CAD build for the part. Positions are in the model's coordinates, mm. A direction names the side the tool comes from. Give positions to 0.01 mm unless a question says otherwise; leave off trailing zeros. Order: outer loops, then holes, each group sorted by start corner. A loop starts at its lowest first (then second) coordinate and runs counter-clockwise, first axis right, second up.
Item 1: Wall check: L1, parallel to X at y = 3.6, z = -24; L2, parallel to X at y = 0.4, z = 17; L3, parallel to X at y = 3.6, z = -6. Give the ranges that are in metal, low to high.
Item 2: Flat gauge pins, fed straight in: P1, Ø2, axis at x = -6, y = 2.5, coming from the +Z side; P2, Ø1, axis at x = -26, y = 0.5, coming from the +Z side (3 decimals). Where does each tip first touch, or does it go through?
Item 3: Band-saw the part on C-C on y = 2.85. Give the cut face in (x, z) (3 decimals), plus the area to 3 significant figures.
Item 4: Band-saw the part on D-D on z = 23.5. Give the cut face in (x, y).
Item 5: Which spindle directions (+Z, -Z, +X, -X, +Y, -Y) get a long thin tool onto all of the face, cutting with end or side? Do faces 5 (the flat face through (-42, 2, 26.725)), 6 (the flat face through (-31, 2, 22.225)), 7 (the flat face through (36, 2, -22.225)), 8 (the flat face through (24, 2, 0)), 9 (the flat face through (0, 2, -26.725)). Say none if no direction does.
Item 6: Two-plate mould, pull along X, no slides. Class faces 1 (the flat face through (-1, 4.5, -6)), 2 (the flat face through (-45, 2, 0)), 3 (the flat face through (40, 2, 24)), 4 (the flat face through (-40, 2, -25)): released by +X, released by -X, zero draft, split by the parting line, or undercut.
Item 7: Band-saw the part on B-B on x = 24. Give the cut face in (y, z) (3 decimals).
Item 8: Band-saw the part on A-A on z = -15. Give the cut face in (x, y), plus the area to 4 significant figures.
```python
from build123d import *

# Parameters (mm, degrees)
SKETCH1_W           = 4.5
SKETCH1_H           = 20
BOSS_EXTRUDE1_DEPTH = 4.5
SKETCH2_W           = 44.2
SKETCH2_H           = 19.225
CUT_EXTRUDE1_DEPTH  = 5.5
SKETCH3_W           = 65
SKETCH3_H           = 4.5
BOSS_EXTRUDE2_DEPTH = 4.5


with BuildPart() as part:
    # Sketch1 → Boss-Extrude1 (new body)
    with BuildSketch(Plane(origin=(0, 0, 0), x_dir=(1, 0, 0), z_dir=(0, 1, 0))):
        Polygon((-40, -22.225), (-40, -26.725), (-45, -26.725), (-45, 26.725), (-40, 26.725), (-40, 22.225), (0, 22.225), (0, -22.225), align=None)
        with Locations((-24.35, 10)):
            Rectangle(SKETCH1_W, SKETCH1_H, mode=Mode.SUBTRACT)
    boss_extrude1 = extrude(amount=BOSS_EXTRUDE1_DEPTH)

    # Mirror1: Boss-Extrude1 across plane
    add(boss_extrude1.mirror(Plane(origin=(0, 4.5, -22.225), x_dir=(0, 0, 1), z_dir=(-1, 0, 0))))

    # Sketch2 → Cut-Extrude1 (cut, through all)
    with BuildSketch(Plane(origin=(0, 4.5, 0), x_dir=(1, 0, 0), z_dir=(0, 1, 0))):
        with Locations((0, -12.6125)):
            Rectangle(SKETCH2_W, SKETCH2_H)
    extrude(amount=-CUT_EXTRUDE1_DEPTH, mode=Mode.SUBTRACT)

    # Sketch3 → Boss-Extrude2 (add)
    with BuildSketch(Plane(origin=(0, 4.5, 0), x_dir=(1, 0, 0), z_dir=(0, 1, 0))):
        with Locations((0, 24.475)):
            Rectangle(SKETCH3_W, SKETCH3_H)
    extrude(amount=-BOSS_EXTRUDE2_DEPTH)


solid = part.part
```
The answers:
1. L1: x = -45 to -40, -32.5 to 32.5, 40 to 45
1. L2: x = -45 to -22.1, 22.1 to 45
1. L3: x = -45 to -26.6, -22.1 to 22.1, 26.6 to 45
2. P1: stops at z = 3
2. P2: stops at z = 22.225
3. outline: (-45, -26.725) - (-40, -26.725) - (-40, -22.225) - (-32.5, -22.225) - (-32.5, -26.725) - (32.5, -26.725) - (32.5, -22.225) - (40, -22.225) - (40, -26.725) - (45, -26.725) - (45, 26.725) - (40, 26.725) - (40, 22.225) - (22.1, 22.225) - (22.1, 3) - (-22.1, 3) - (-22.1, 22.225) - (-40, 22.225) - (-40, 26.725) - (-45, 26.725) - close; hole (-26.6, -20) - (-22.1, -20) - (-22.1, 0) - (-26.6, 0) - close; hole (22.1, -20) - (26.6, -20) - (26.6, 0) - (22.1, 0) - close
3. area: 3,350 mm2
4. outline: (-45, 0) - (-40, 0) - (-40, 4.5) - (-45, 4.5) - close; (40, 0) - (45, 0) - (45, 4.5) - (40, 4.5) - close
5. face 5: +Z, +X, -X, +Y, -Y
5. face 6: +Z, +Y, -Y
5. face 7: -Z, +Y, -Y
5. face 8: +Y, -Y
5. face 9: -Z, +X, -X, +Y, -Y
6. face 1: zero draft
6. face 2: released by -X
6. face 3: undercut
6. face 4: undercut
7. outline: (0, -26.725) - (4.5, -26.725) - (4.5, -20) - (0, -20) - close; (0, 0) - (4.5, 0) - (4.5, 22.225) - (0, 22.225) - close
8. outline: (-45, 0) - (-26.6, 0) - (-26.6, 4.5) - (-45, 4.5) - close; (-22.1, 0) - (22.1, 0) - (22.1, 4.5) - (-22.1, 4.5) - close; (26.6, 0) - (45, 0) - (45, 4.5) - (26.6, 4.5) - close
8. area: 364.5 mm2
